The model under review builds one solid part; all positions refer to its coordinate system, in mm. Give positions to 0.01 mm unless a question says otherwise; leave off trailing zeros. Loops run counter-clockwise (first coordinate to the right, second up) from the corner with the lowest first, then second, coordinate; pieces in that order, holes last. Notation, with made-up numbers: M -37.5,-7 L 19.5,-7 A23 cw 19.5,6 Z; hole C 76,53.5 d1. An arc over 180 degrees is marked long. Write item = value, one per line. Start each with the question number.
1. We need section D-D on x = 4.5. Give the boundary of the cut face in (y, z).
2. For pin 1 (5 mm diameter, centred on y = 4, z = -3.5, fed in from -X); pin 2 (1 mm diameter, centred on x = 0, z = 1, fed in from -Y) (3 decimals); pin 3 (3 mm diameter, centred on x = 0.5, y = 4.5, fed in from -Z); pin 4 (1.5 mm diameter, centred on x = 2, y = -1, fed in from +Z), all flat-tipped, find the tip position at first contact; note any pin that passes through.
3. We need section A-A on x = 0. Give the boundary of the cut face in (y, z), then the cut area to 3 significant figures.
4. We need section C-C on y = 3.5. Give the boundary of the cut face in (x, z).
5. We need section B-B on z = 0. Give the boundary of the cut face in (x, y), then the cut area to 3 significant figures.
6. Wall thickness on line 1 along Z through (x, y) = (0, 4); line 2 along Y through (x, z) = (4.5, -1.75); line 3 along X through (y, z) = (-2.5, -0.75): over which ranges is each line inside the solid? List them lowest first. Write a range as from..to.
7. Draft analysis for pull direction X (two halves, no side actions). For faces 1 (the face through (-3.905, 1.819, -0.867)), 2 (the face through (-2, -7.15, 2)), 3 (the face through (1.18, 0.1, 2.26)), state which applies: pulls with the +X half, pulls with the -X half, needs draft (parallel to the pull), parting line crosses it, or undercut.
from build123d import *

# Parameters (mm, degrees)
SKETCH_1_R              = 4
EXTRUDE_1_DEPTH         = 7.15
SKETCH_2_W              = 1
SKETCH_2_H              = 4
CHAMFER_1_SIZE          = 0.5
HOLE_WIZARD_5_1_5_1_1_D = 5.1


with BuildPart() as part:
    # 草图1 → 凸台-拉伸1 (new, symmetric)
    with BuildSketch(Plane(origin=(0, 0, 0), x_dir=(1, 0, 0), z_dir=(0, 1, 0))):
        with Locations(Location((0, 0, 0), (0, 0, 270))):
            Circle(SKETCH_1_R)
    extrude(amount=EXTRUDE_1_DEPTH, both=True)

    # 草图2 → 旋转1 (revolve)
    with BuildSketch(Plane.XY, mode=Mode.PRIVATE) as revolve_1_sk:
        with Locations((4.5, -5.15)):
            Rectangle(SKETCH_2_W, SKETCH_2_H)
    revolve(revolve_1_sk.sketch.rotate(Axis((0, 7.15, 0), (0, -1, 0)), 270), axis=Axis((0, 7.15, 0), (0, -1, 0)))

    # 倒角1
    chamfer_1_edges = [part.edges().sort_by_distance(p)[0] for p in [
        (0, 7.15, -4),
    ]]
    chamfer(chamfer_1_edges, length=CHAMFER_1_SIZE)

    # Ø5.1 (5.1) 直径孔1 (through all)
    with Locations(Plane(origin=(0, -7.15, 0), x_dir=(-1, 0, 0), z_dir=(0, -1, 0))):
        with Locations((0, 0)):
            Hole(HOLE_WIZARD_5_1_5_1_1_D / 2)


solid = part.part
Final values:
q1.outline = M -7.15,-2.18 L -3.15,-2.18 L -3.15,2.18 L -7.15,2.18 Z
q2.pin_1 = -3.87
q2.pin_2 = through
q2.pin_3 = -4
q2.pin_4 = 3.8
q3.outline = M -7.15,-5 L -3.15,-5 L -3.15,-4 L 6.65,-4 L 7.15,-3.5 L 7.15,-2.55 L -7.15,-2.55 Z; M -7.15,2.55 L 7.15,2.55 L 7.15,3.5 L 6.65,4 L -3.15,4 L -3.15,5 L -7.15,5 Z
q3.area = 49.2 mm²
q4.outline = C 0,0 d8; hole C 0,0 d5.1
q5.outline = M -5,-7.15 L -2.55,-7.15 L -2.55,7.15 L -3.5,7.15 L -4,6.65 L -4,-3.15 L -5,-3.15 Z; M 2.55,-7.15 L 5,-7.15 L 5,-3.15 L 4,-3.15 L 4,6.65 L 3.5,7.15 L 2.55,7.15 Z
q5.area = 49.2 mm²
q6.line_1 = -4..-2.55, 2.55..4
q6.line_2 = -7.15..-3.15
q6.line_3 = -3.93..-2.44, 2.44..3.93
q7.face_1 = parting line crosses it
q7.face_2 = needs draft
q7.face_3 = undercut
